The figure shows three views and two pictorial views of one solid part (mm, origin at its lowest corner). Answer the questions. Give positions to 0.01 mm unless a question says otherwise; leave off trailing zeros. Order: outer loops, then holes, each group sorted by start corner. A loop starts at its lowest first (then second) coordinate and runs counter-clockwise, first axis right, second up. Notation, with made-up numbers: (4.5, 84.5) - (47.5, 84.5) arc R31 cw to (47.5, 112.5) - close; hole circle Ø10 at (-3.75, 14.5). An arc over 180 degrees is marked (long way). Answer as CSV lines item,"result". Start each with the question number.
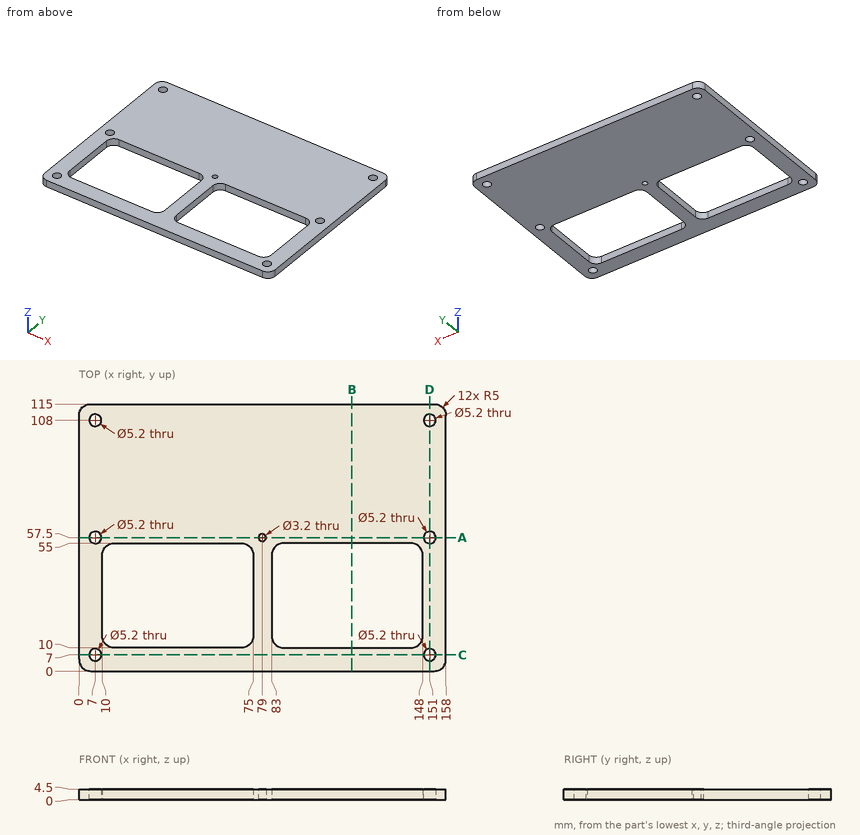
(1) Straight lines are drawn through the part: line 1 (Y direction, x = 7, z = 2.9); line 2 (X direction, y = 32.5, z = 1.3); line 3 (X direction, y = 54.5, z = 3.45). For each, find the intervals that lie inside material, in ascending order. Write a range as [from, to].
(2) Section C-C, the plane y = 7 is taken. Write down the section's boundary in (x, z).
(3) Section A-A, the plane y = 57.5 is taken. Write down the section's boundary in (x, z), and give its area (3 significant figures).
(4) Section B-B, the plane x = 117.5 is taken. Write down the section's boundary in (y, z).
(5) Section D-D, the plane x = 151 is taken. Write down the section's boundary in (y, z), and give its area (3 significant figures).
Checks:
1,line 1,"y = [0, 4.4], [9.6, 54.9], [60.1, 105.4], [110.6, 115]"
1,line 2,"x = [0, 10], [75, 83], [148, 158]"
1,line 3,"x = [0, 12.82], [72.18, 85.82], [145.18, 158]"
2,outline,"(0, 0) - (4.4, 0) - (4.4, 4.5) - (0, 4.5) - close; (9.6, 0) - (148.4, 0) - (148.4, 4.5) - (9.6, 4.5) - close; (153.6, 0) - (158, 0) - (158, 4.5) - (153.6, 4.5) - close"
3,outline,"(0, 0) - (4.4, 0) - (4.4, 4.5) - (0, 4.5) - close; (9.6, 0) - (77.4, 0) - (77.4, 4.5) - (9.6, 4.5) - close; (80.6, 0) - (148.4, 0) - (148.4, 4.5) - (80.6, 4.5) - close; (153.6, 0) - (158, 0) - (158, 4.5) - (153.6, 4.5) - close"
3,area,"650 mm²"
4,outline,"(0, 0) - (10, 0) - (10, 4.5) - (0, 4.5) - close; (55, 0) - (115, 0) - (115, 4.5) - (55, 4.5) - close"
5,outline,"(0, 0) - (4.4, 0) - (4.4, 4.5) - (0, 4.5) - close; (9.6, 0) - (54.9, 0) - (54.9, 4.5) - (9.6, 4.5) - close; (60.1, 0) - (105.4, 0) - (105.4, 4.5) - (60.1, 4.5) - close; (110.6, 0) - (115, 0) - (115, 4.5) - (110.6, 4.5) - close"
5,area,"447 mm²"
